from build123d import *

# Parameters (mm, degrees)
F0_R     = 27.305
F1_DEPTH = 6.35
F2_R     = 3.937
F3_DEPTH = 12.7
F0_R_2   = 31.75
F4_DEPTH = 6.3754
F5_R     = 1.27


# Not quite as in the source:
# - a fillet or chamfer that OpenCascade refuses, or shapes differently, is made with other operations: its cross-section is extruded or revolved along the edge and cut away or added


with BuildPart() as f1:
    # F0 (on Top) → F1 (new body, symmetric)
    with BuildSketch(Plane.XY):
        Circle(F0_R)
    extrude(amount=F1_DEPTH, both=True)

    # F2 (on Top) → F3 (cut, symmetric)
    with BuildSketch(Plane.XY):
        Circle(F2_R)
    extrude(amount=F3_DEPTH, both=True, mode=Mode.SUBTRACT)

    # F0 (on Top) → F4 (join)
    with BuildSketch(Plane.XY):
        Circle(F0_R_2)
        Circle(F0_R, mode=Mode.SUBTRACT)
    extrude(amount=F4_DEPTH)

    # F5
    f5_edges = [f1.edges().sort_by_distance(p)[0] for p in [
        (-27.305, 0, -6.35),
    ]]
    fillet(f5_edges, radius=F5_R)

    # F6: fillet of radius 5.08 on 1 edges, made by hand

    # F6_s1 → F6_t2 (revolve, cut)
    with BuildSketch(Plane.XZ):
        with BuildLine():
            ThreePointArc((31.75, 1.3352437524), (30.48, 4.6953479175), (27.305, 6.3754))
            Line((27.305, 6.3754), (31.75, 6.3754))
            Line((31.75, 6.3754), (31.75, 1.3352437524))
        make_face()
    revolve(axis=Axis((0, 0, 6.3754), (0, 0, 1)), mode=Mode.SUBTRACT)


solid = f1.part
Can you work these out from the model? Positions are in its coordinate system, mm. Give positions to 0.01 mm unless a question says otherwise; leave off trailing zeros. Loops run counter-clockwise (first coordinate to the right, second up) from the corner with the lowest first, then second, coordinate; pieces in that order, holes last. Notation, with made-up numbers: M 51.5,1.25 L 81.5,1.25 A10 cw 81.5,17.25 Z; hole C 86.25,11.5 d7. An arc over 180 degrees is marked long. One line per item, written item: value. Start each with the question number.
1) If we section it at C-C, the plane z = -2.25: Write out the boundary of the cut face in (x, y) (3 decimals).
2) If we section it at D-D, the plane z = 3: Write out the boundary of the cut face in (x, y), and give its area (3 significant figures).
3) If I drill on line 1 (Y direction, x = 0, z = 1); line 2 (Z direction, x = -7, y = -1); line 3 (Z direction, x = -26, y = 9), over which ranges is the centre line in solid material (lowest first)? Write a range as [from, to].
4) Thinking about a two-plate mould opening in Y: for faces 1 (the face through (-6.883, -30.995, 0.658)), 2 (the face through (14, 24, 0)), 3 (the face through (-0.853, -3.843, 0.089)), which applies, +Y half, -Y half, draft (parallel to the pull), parting line (faces both ways), or undercut?
5) I'm going to push flat-ended pins straight in: pin 1 (2 mm diameter, centred on y = -15.5, z = 3.5, fed in from +X); pin 2 (6 mm diameter, centred on x = -11, z = -1.5, fed in from +Y); pin 3 (4 mm diameter, centred on x = -12, z = -1.5, fed in from -Y). Where does each tip first touch, or does it pass through?
6) If we section it at A-A, the plane x = 0: Write out the boundary of the cut face in (y, z) (3 decimals).
Completed:
1. outline: C 0,0 d54.61; hole C 0,0 d7.874
2. outline: C 0,0 d62.94; hole C 0,0 d7.87
2. area: 3,060 mm^2
3. line 1: y = [-31.75, -3.94], [3.94, 31.75]
3. line 2: z = [-6.35, 6.35]
3. line 3: z = [0, 6.34]
4. face 1: parting line
4. face 2: draft
4. face 3: undercut
5. pin 1: stops at x = 27.86
5. pin 2: stops at y = 30.62
5. pin 3: stops at y = -29.9
6. outline: M -31.75,0 L -27.305,0 L -27.305,-5.08 A1.27 ccw -26.035,-6.35 L -3.937,-6.35 L -3.937,6.35 L -27.305,6.35 L -27.305,6.375 A5.08 ccw -31.75,1.335 Z; M 3.937,-6.35 L 26.035,-6.35 A1.27 ccw 27.305,-5.08 L 27.305,0 L 31.75,0 L 31.75,1.335 A5.08 ccw 27.305,6.375 L 27.305,6.35 L 3.937,6.35 Z
